Could you check a few things on this model? Use its own coordinates, in mm. A direction names the side the tool comes from. Round coordinates to 2 decimals unless told otherwise and drop trailing zeros. Loops run counter-clockwise (first coordinate to the right, second up) from the corner with the lowest first, then second, coordinate; pieces in that order, holes last. Notation, with made-up numbers: (33.5, 52) -> (90.5, 52) arc R27 cw to (90.5, 90) -> close; hole circle Ø1 at (63, 83). An arc over 180 degrees is marked (long way). Use CSV: the item, a comma, the result in double quotes. Start each with the question number.
```python
from build123d import *

# Parameters (mm, degrees)
SKETCH1_W                 = 114.3
SKETCH1_H                 = 177.8
SKETCH1_W_2               = 101.6
SKETCH1_H_2               = 165.1
BOSS_EXTRUDE1_DEPTH       = 4.7625
SKETCH2_W                 = 12.38677804
SKETCH2_H                 = 4.7625
SKETCH2_W_2               = 12.7
BOSS_EXTRUDE2_DEPTH       = 4.7625
SKETCH3_W                 = 12.7
SKETCH3_H                 = 4.7625
BOSS_EXTRUDE3_DEPTH       = 4.7625
FILLET1_R                 = 2.54
SKETCH4_W                 = 114.3
SKETCH4_H                 = 12.7
BOSS_EXTRUDE4_DEPTH       = 4.7625
F_6_CLEARANCE_HOLE1_D     = 3.7973
F_6_CLEARANCE_HOLE1_DEPTH = 25.4
F_6_CLEARANCE_HOLE1_TIP   = 1.140824014
FILLET2_R                 = 2.54


with BuildPart() as part:
    # Sketch1 → Boss-Extrude1 (new body)
    with BuildSketch(Plane(origin=(0, 0, 0), x_dir=(1, 0, 0), z_dir=(0, 1, 0))):
        Rectangle(SKETCH1_W, SKETCH1_H)
        Rectangle(SKETCH1_W_2, SKETCH1_H_2, mode=Mode.SUBTRACT)
    extrude(amount=BOSS_EXTRUDE1_DEPTH)

    # Sketch2 → Boss-Extrude2 (add)
    with BuildSketch(Plane.XY.offset(88.9)):
        with Locations((-38.1, 2.38125)):
            Rectangle(SKETCH2_W, SKETCH2_H)
        with Locations((12.7, 2.38125)):
            Rectangle(SKETCH2_W_2, SKETCH2_H)
    extrude(amount=BOSS_EXTRUDE2_DEPTH)

    # Sketch3 → Boss-Extrude3 (add)
    with BuildSketch(Plane(origin=(0, 0, -88.9), x_dir=(-1, 0, 0), z_dir=(0, 0, -1))):
        with Locations((-38.1, 2.38125)):
            Rectangle(SKETCH3_W, SKETCH3_H)
        with Locations((12.7, 2.38125)):
            Rectangle(SKETCH3_W, SKETCH3_H)
    extrude(amount=BOSS_EXTRUDE3_DEPTH)

    # Fillet1
    fillet1_edges = [part.edges().sort_by_distance(p)[0] for p in [
        (50.8, 2.38125, 82.55),
        (50.8, 2.38125, -82.55),
        (-50.8, 2.38125, -82.55),
        (-50.8, 2.38125, 82.55),
    ]]
    fillet(fillet1_edges, radius=FILLET1_R)

    # Sketch4 → Boss-Extrude4 (add)
    with BuildSketch(Plane(origin=(0, 4.7625, 0), x_dir=(1, 0, 0), z_dir=(0, 1, 0))):
        with Locations((0, 46.149999902)):
            Rectangle(SKETCH4_W, SKETCH4_H)
        with Locations((0, -58.849999902)):
            Rectangle(SKETCH4_W, SKETCH4_H)
    extrude(amount=-BOSS_EXTRUDE4_DEPTH)

    # #6 Clearance Hole1
    with Locations(Plane(origin=(0, 4.7625, 0), x_dir=(-1, 0, 0), z_dir=(0, 1, 0))):
        with Locations((52.5, -46.149999902), (-52.5, -46.149999902), (52.5, 58.849999902), (-52.5, 58.849999902)):
            Hole(F_6_CLEARANCE_HOLE1_D / 2, depth=F_6_CLEARANCE_HOLE1_DEPTH)
            with Locations((0, 0, -(F_6_CLEARANCE_HOLE1_DEPTH + F_6_CLEARANCE_HOLE1_TIP / 2))):  # 118° drill point
                Cone(0, F_6_CLEARANCE_HOLE1_D / 2, F_6_CLEARANCE_HOLE1_TIP, mode=Mode.SUBTRACT)

    # Fillet2
    fillet2_edges = [part.edges().sort_by_distance(p)[0] for p in [
        (-50.8, 2.38125, -39.799999902),
        (-50.8, 2.38125, -52.499999902),
        (50.8, 2.38125, -52.499999902),
        (50.8, 2.38125, -39.799999902),
        (-50.8, 2.38125, 65.199999902),
        (-50.8, 2.38125, 52.499999902),
        (50.8, 2.38125, 52.499999902),
        (50.8, 2.38125, 65.199999902),
    ]]
    fillet(fillet2_edges, radius=FILLET2_R)


solid = part.part
```
1. For faces 1 (the face through (50.8, 2, 74)), 2 (the face through (-13, 2, 88.9)), 3 (the face through (-44.293, 2, 91)), 4 (the face through (-6.35, 2, -91)), which set-ups out of +Z, -Z, +X, -X, +Y, -Y let a thin tool reach every point of the face, with its end or its side?
2. Suppose I cut it at A-A (z = 18.5). List the corners of the cut face in (x, y) for me, then the cut area to 3 significant figures.
3. Suppose I cut it at B-B (x = -2.5). List the corners of the cut face in (y, z) for me, then the cut area to 3 significant figures.
4. Suppose I cut it at D-D (y = 3.1). State how many separate pieces and enclosed holes the cut face has, then the cut area to 3 significant figures.
5. If I drill on L1, parallel to X at y = 2.55, z = 58.85; L2, parallel to Z at x = 33, y = 2.4; L3, parallel to Z at x = -52.5, y = 3.05, over which ranges is the centre line in solid material (lowest first)?
6. Will these pins go through, and if not, where does the flat tip stop? pin 1 (2.5 mm diameter, centred on x = -15.5, y = 3.5, fed in from +Z); pin 2 (2.5 mm diameter, centred on x = -23, y = 3.5, fed in from -Z); pin 3 (1.4 mm diameter, centred on y = 2, z = 91, fed in from -X).
7. We'd pull the mould along X, two halves only. Please class faces 5 (the face through (38, 2, 88.9)), 6 (the face through (-19.05, 2, -91)), 7 (the face through (-50.8, 2, -67)): pulls with the +X half, pulls with the -X half, needs draft (parallel to the pull), parting line crosses it, or undercut.
8. Suppose I cut it at C-C (z = -46.15). List the corners of the cut face in (x, y) for me, then the cut area to 3 significant figures.
Geometry check:
1,face 1,"+Y, -Y"
1,face 2,"+Z, +Y, -Y"
1,face 3,"+Z, -X, +Y, -Y"
1,face 4,"-Z, +Y, -Y"
2,outline,"(-57.15, 0) -> (-50.8, 0) -> (-50.8, 4.76) -> (-57.15, 4.76) -> close; (50.8, 0) -> (57.15, 0) -> (57.15, 4.76) -> (50.8, 4.76) -> close"
2,area,"60.5 mm²"
3,outline,"(0, -88.9) -> (4.76, -88.9) -> (4.76, -82.55) -> (0, -82.55) -> close; (0, -52.5) -> (4.76, -52.5) -> (4.76, -39.8) -> (0, -39.8) -> close; (0, 52.5) -> (4.76, 52.5) -> (4.76, 65.2) -> (0, 65.2) -> close; (0, 82.55) -> (4.76, 82.55) -> (4.76, 88.9) -> (0, 88.9) -> close"
3,area,"181 mm²"
4,separate pieces,"1"
4,enclosed holes,"7"
4,area,"6,340 mm²"
5,L1,"x = -57.15 to -54.4, -50.6 to 50.6, 54.4 to 57.15"
5,L2,"z = -93.66 to -82.55, -52.5 to -39.8, 52.5 to 65.2, 82.55 to 88.9"
5,L3,"z = -88.9 to -48.05, -44.25 to 56.95, 60.75 to 88.9"
6,pin 1,"stops at z = 88.9"
6,pin 2,"stops at z = -88.9"
6,pin 3,"stops at x = -44.29"
7,face 5,"needs draft"
7,face 6,"pulls with the -X half"
7,face 7,"undercut"
8,outline,"(-57.15, 0) -> (-54.4, 0) -> (-54.4, 4.76) -> (-57.15, 4.76) -> close; (-50.6, 0) -> (50.6, 0) -> (50.6, 4.76) -> (-50.6, 4.76) -> close; (54.4, 0) -> (57.15, 0) -> (57.15, 4.76) -> (54.4, 4.76) -> close"
8,area,"508 mm²"
